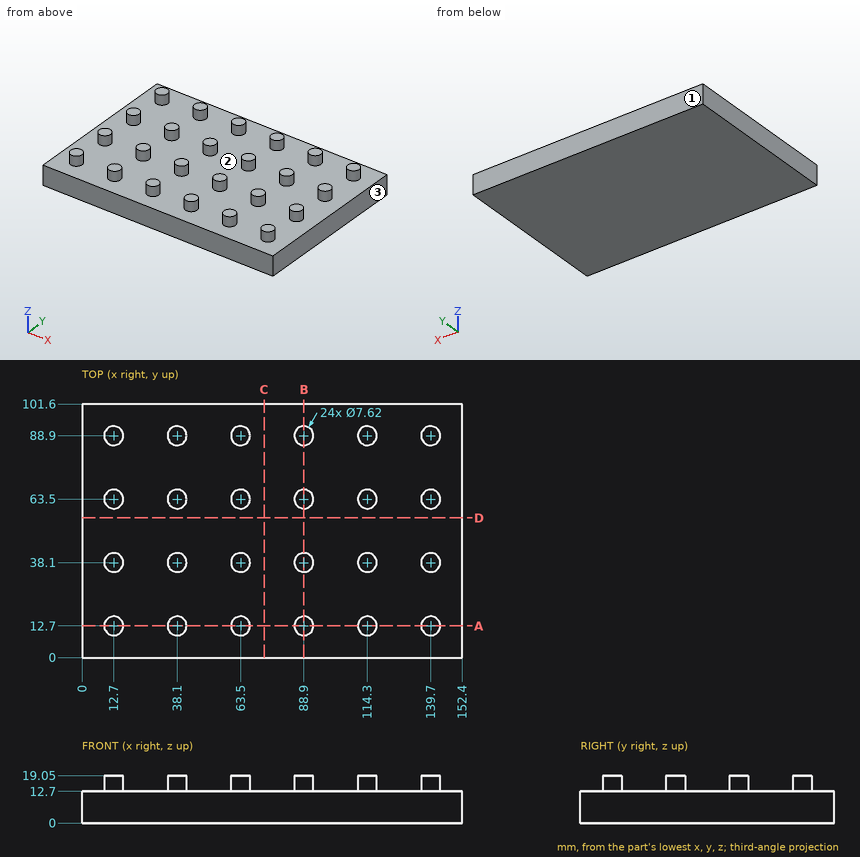
Input: dimensioned drawing with shaded views. Units: mm. Origin: part minimum x, y, z. Coordinates: 2 decimals unless noted, no trailing zeros. Loops run counter-clockwise (first coordinate to the right, second up) from the corner with the lowest first, then second, coordinate; pieces in that order, holes last. Notation, with made-up numbers: (-23.75, 65) -> (6.25, 65) arc R15 ccw to (6.25, 90) -> close; hole circle Ø4 at (-24, 43.25). An arc over 180 degrees is marked (long way). Use a Markdown table: item, result. Add a question column.
(1) Section query A-A, the plane y = 12.7. Return loops of the section in (x, z), plus the area to 3 significant figures.
(2) Line query: line 1 along X through (y, z) = (88, 16); line 2 along Y through (x, z) = (12, 17.75); line 3 along Z through (x, y) = (84.5, 76.5). Output: solid intervals per line, ascending.
(3) Section query D-D, the plane y = 56. Return loops of the section in (x, z), plus the area to 3 significant figures.
(4) Pin query (flat end, axial travel): pin 1 Ø8 at (x, y) = (132, 70.5) entering from +Z; pin 2 Ø1 at (y, z) = (56, 13.5) entering from +X. Return the tip coordinate at first contact, or that it passes through.
(5) Mould query, pull axis X, two halves, no side actions, for the marked faces 1, 2 and 3. Classes: pulls with the +X half, pulls with the -X half, needs draft (parallel to the pull), parting line crosses it, or undercut.
(6) Section query B-B, the plane x = 88.9. Return loops of the section in (y, z), plus the area to 3 significant figures.
(7) Section query C-C, the plane x = 73. Return loops of the section in (y, z).
Answer:
| question | item | result |
|---|---|---|
| 1 | outline | (0, 0) -> (152.4, 0) -> (152.4, 12.7) -> (143.51, 12.7) -> (143.51, 19.05) -> (135.89, 19.05) -> (135.89, 12.7) -> (118.11, 12.7) -> (118.11, 19.05) -> (110.49, 19.05) -> (110.49, 12.7) -> (92.71, 12.7) -> (92.71, 19.05) -> (85.09, 19.05) -> (85.09, 12.7) -> (67.31, 12.7) -> (67.31, 19.05) -> (59.69, 19.05) -> (59.69, 12.7) -> (41.91, 12.7) -> (41.91, 19.05) -> (34.29, 19.05) -> (34.29, 12.7) -> (16.51, 12.7) -> (16.51, 19.05) -> (8.89, 19.05) -> (8.89, 12.7) -> (0, 12.7) -> close |
| 1 | area | 2,230 mm^2 |
| 2 | line 1 | x = 9 to 16.4, 34.4 to 41.8, 59.8 to 67.2, 85.2 to 92.6, 110.6 to 118, 136 to 143.4 |
| 2 | line 2 | y = 8.95 to 16.45, 34.35 to 41.85, 59.75 to 67.25, 85.15 to 92.65 |
| 2 | line 3 | z = 0 to 12.7 |
| 3 | outline | (0, 0) -> (152.4, 0) -> (152.4, 12.7) -> (0, 12.7) -> close |
| 3 | area | 1,940 mm^2 |
| 4 | pin 1 | stops at z = 12.7 |
| 4 | pin 2 | passes through |
| 5 | face 1 | needs draft |
| 5 | face 2 | undercut |
| 5 | face 3 | pulls with the +X half |
| 6 | outline | (0, 0) -> (101.6, 0) -> (101.6, 12.7) -> (92.71, 12.7) -> (92.71, 19.05) -> (85.09, 19.05) -> (85.09, 12.7) -> (67.31, 12.7) -> (67.31, 19.05) -> (59.69, 19.05) -> (59.69, 12.7) -> (41.91, 12.7) -> (41.91, 19.05) -> (34.29, 19.05) -> (34.29, 12.7) -> (16.51, 12.7) -> (16.51, 19.05) -> (8.89, 19.05) -> (8.89, 12.7) -> (0, 12.7) -> close |
| 6 | area | 1,480 mm^2 |
| 7 | outline | (0, 0) -> (101.6, 0) -> (101.6, 12.7) -> (0, 12.7) -> close |
